Geometry check sheet. Reference: drawing and pictorial views, mm from the part's lowest x, y, z. A direction names the side the tool comes from. Coordinates: 2 decimals unless noted, no trailing zeros. Loops run counter-clockwise (first coordinate to the right, second up) from the corner with the lowest first, then second, coordinate; pieces in that order, holes last. Notation, with made-up numbers: (41, 46.5) -> (62, 46.5) arc R28 cw to (62, 76.5) -> close; hole circle Ø10 at (46, 81.5). An arc over 180 degrees is marked (long way). Use CSV: the item, a comma, the result in double quotes.
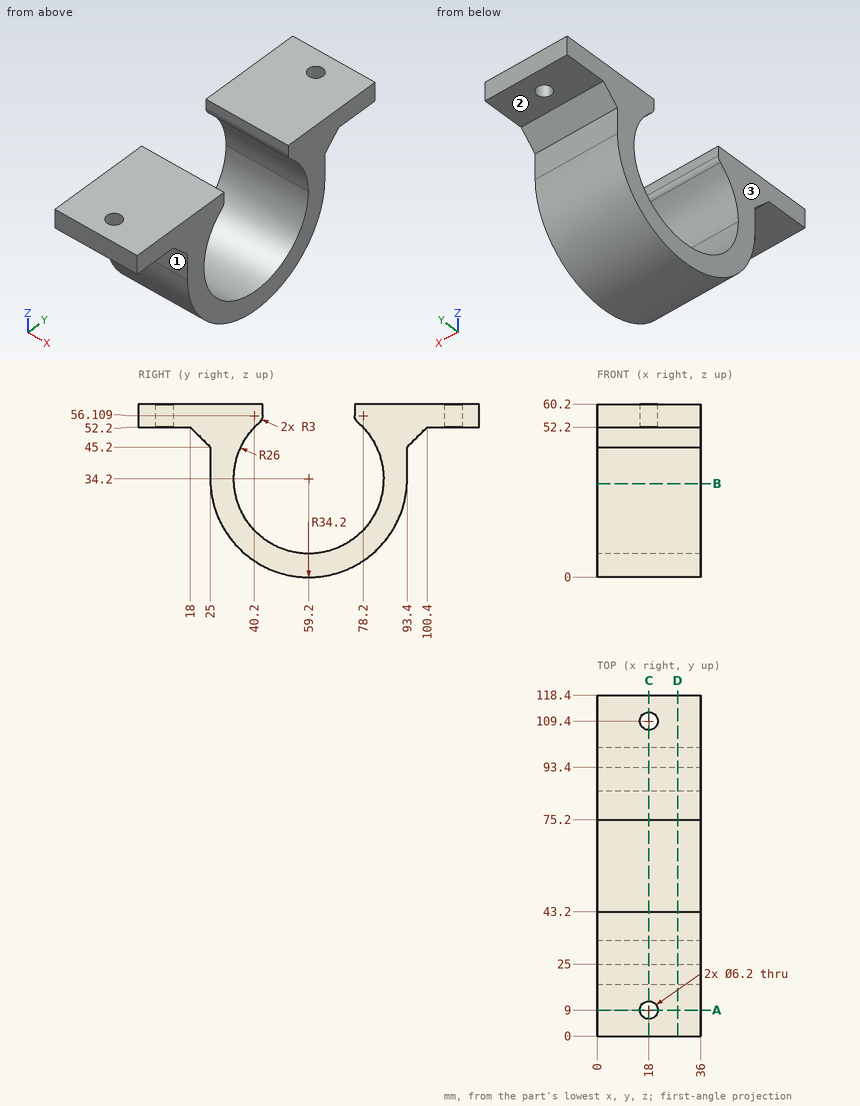
1) Access from +Z, -Z, +X, -X, +Y, -Y to the whole of each face (thin tool, end or side, straight path). Record for the marked faces 1, 2 and 3.
Answer below:
face 1,"-Z, +X, -X, -Y"
face 2,"-Z, +X, -X, +Y"
face 3,"+Z, -Z, -X, +Y, -Y"
2) Cross-section at A-A on y = 9. Record the boundary of the cut face in (x, z).
Answer below:
outline,"(0, 52.2) -> (14.9, 52.2) -> (14.9, 60.2) -> (0, 60.2) -> close; (21.1, 52.2) -> (36, 52.2) -> (36, 60.2) -> (21.1, 60.2) -> close"
3) Thickness scan on line 1 along Y through (x, z) = (18, 57); line 2 along X through (y, z) = (9, 57); line 3 along Y through (x, z) = (18, 55). Record the ranges inside material, lowest first. Write a range as from..to.
Answer below:
line 1,"y = 0..5.9, 12.1..43.2, 75.2..106.3, 112.5..118.4"
line 2,"x = 0..14.9, 21.1..36"
line 3,"y = 0..5.9, 12.1..42.99, 75.41..106.3, 112.5..118.4"
4) Cross-section at B-B on z = 32.5. Record the boundary of the cut face in (x, y).
Answer below:
outline,"(0, 25.04) -> (36, 25.04) -> (36, 33.26) -> (0, 33.26) -> close; (0, 85.14) -> (36, 85.14) -> (36, 93.36) -> (0, 93.36) -> close"
5) Go/stop test with flat-tipped pins: pin 1 Ø1.5 at (x, z) = (31.5, 39.5) entering from +Y; pin 2 Ø20 at (x, y) = (24, 110.5) entering from -Z; pin 3 Ø4 at (x, z) = (20.5, 14.5) entering from +Y. Record where each tip stops, or that it passes through.
Answer below:
pin 1,"stops at y = 93.4"
pin 2,"stops at z = 52.2"
pin 3,"stops at y = 88.46"
6) Cross-section at C-C on x = 18. Record the boundary of the cut face in (y, z), and give its area (3 significant figures).
Answer below:
outline,"(0, 52.2) -> (5.9, 52.2) -> (5.9, 60.2) -> (0, 60.2) -> close; (12.1, 52.2) -> (18, 52.2) -> (25, 45.2) -> (25, 34.2) arc R34.2 ccw to (93.4, 34.2) -> (93.4, 45.2) -> (100.4, 52.2) -> (106.3, 52.2) -> (106.3, 60.2) -> (75.2, 60.2) -> (75.2, 56.11) arc R3 ccw to (76.23, 53.84) arc R26 cw to (85.2, 34.2) arc R26 cw to (33.2, 34.2) arc R26 cw to (42.17, 53.84) arc R3 ccw to (43.2, 56.11) -> (43.2, 60.2) -> (12.1, 60.2) -> close; (112.5, 52.2) -> (118.4, 52.2) -> (118.4, 60.2) -> (112.5, 60.2) -> close"
area,"1,790 mm²"
7) Cross-section at D-D on x = 28. Record the boundary of the cut face in (y, z).
Answer below:
outline,"(0, 52.2) -> (18, 52.2) -> (25, 45.2) -> (25, 34.2) arc R34.2 ccw to (93.4, 34.2) -> (93.4, 45.2) -> (100.4, 52.2) -> (118.4, 52.2) -> (118.4, 60.2) -> (75.2, 60.2) -> (75.2, 56.11) arc R3 ccw to (76.23, 53.84) arc R26 cw to (85.2, 34.2) arc R26 cw to (33.2, 34.2) arc R26 cw to (42.17, 53.84) arc R3 ccw to (43.2, 56.11) -> (43.2, 60.2) -> (0, 60.2) -> close"
